Could you check a few things on this model? Use its own coordinates, in mm. A direction names the side the tool comes from. Coordinates: 2 decimals unless noted, no trailing zeros. Order: outer loops, then holes, each group sorted by start corner. A loop starts at its lowest first (then second) coordinate and runs counter-clockwise, first axis right, second up. Notation, with made-up numbers: (-24.75, 29) -> (5.25, 29) arc R18 ccw to (5.25, 46) -> close; hole circle Ø8 at (33.5, 62.5). An arc over 180 degrees is marked (long way). Use a Markdown table: item, result. Add a question column.
1) If we section it at A-A (y = -19.5): Give the number of separate pieces and of enclosed holes in the cut face, plus the area to 3 significant figures.
2) Will these pins go through, and if not, where does the flat tip stop? pin 1 Ø7.5 at (y, z) = (-16.5, 23) entering from -X; pin 2 Ø6 at (x, y) = (-173, -19.5) entering from +Z; pin 3 Ø7.5 at (y, z) = (-20, 35.5) entering from +X.
3) Thinking about a two-plate mould opening in X: for faces 4 (the cylindrical face through (-177.996, -19.312, 9.535)), 5 (the flat face through (-194, -18, 12)), 6 (the flat face through (-178.5, -20, 31)), which applies, +X half, -X half, draft (parallel to the pull), parting line (faces both ways), or undercut?
4) If I drill on L1, parallel to Y at x = -180, z = 45; L2, parallel to X at y = -24.5, z = 24; L3, parallel to Y at x = -173, z = 8, over which ranges is the centre line in solid material (lowest first)? Write a range as [from, to].
5) If we section it at C-C (x = -173): Write out the boundary of the cut face in (y, z), plus the area to 3 significant figures.
6) If we section it at D-D (z = 38): Write out the boundary of the cut face in (x, y).
7) If we section it at B-B (z = 45): Write out the boundary of the cut face in (x, y).
8) Which directions (+Z, -Z, +X, -X, +Y, -Y) give clear straight access to the entire face, cutting with the end or side of a thin tool? Please do faces 1 (the cylindrical face through (-181.458, -19.379, 47.747)), 2 (the flat face through (-171, -17, 7)), 3 (the flat face through (-187.5, -20, 35)).
```python
from build123d import *

# Parameters (mm, degrees)
SKETCH_1_W                   = 15
SKETCH_1_H                   = 15
EXTRUDE_1_DEPTH              = 50
SKETCH_2_W                   = 3
SKETCH_2_H                   = 15
CUT_EXTRUDE_1_DEPTH          = 30
SKETCH_3_W                   = 10
SKETCH_3_H                   = 15
EXTRUDE_2_DEPTH              = 12
HOLE_WIZARD_M5_2_D           = 5.3
HOLE_WIZARD_M5_2_CBORE_D     = 10
HOLE_WIZARD_M5_2_CBORE_DEPTH = 5
CUT_EXTRUDE_2_REACH          = 64.081
SKETCH_8_R                   = 2.75
M5X0_8_1_D                   = 4.2


with BuildPart() as part:
    # 草图1 → 凸台-拉伸1 (new body)
    with BuildSketch(Plane.XY):
        with Locations((-186, -19.5)):
            Rectangle(SKETCH_1_W, SKETCH_1_H)
    extrude(amount=EXTRUDE_1_DEPTH)

    # 草图2 → 切除-拉伸1 (cut)
    with BuildSketch(Plane.XY.offset(50)):
        with Locations((-186, -19.5)):
            Rectangle(SKETCH_2_W, SKETCH_2_H)
    extrude(amount=-CUT_EXTRUDE_1_DEPTH, mode=Mode.SUBTRACT)

    # 草图3 → 凸台-拉伸2 (add)
    with BuildSketch(Plane(origin=(0, 0, 0), x_dir=(-1, 0, 0), z_dir=(0, 0, -1))):
        with Locations((173.5, -19.5)):
            Rectangle(SKETCH_3_W, SKETCH_3_H)
        with Locations((198.5, -19.5)):
            Rectangle(SKETCH_3_W, SKETCH_3_H)
    extrude(amount=-EXTRUDE_2_DEPTH)

    # M5 凹头盖螺钉的柱形沉头孔2 (through all)
    with Locations(Plane.XY.offset(12)):
        with Locations((-199, -19.5), (-173, -19.5)):
            CounterBoreHole(HOLE_WIZARD_M5_2_D / 2, HOLE_WIZARD_M5_2_CBORE_D / 2, HOLE_WIZARD_M5_2_CBORE_DEPTH)

    # 草图8 → 切除-拉伸2 (cut, up to next)
    with BuildSketch(Plane(origin=(-178.5, 0, 0), x_dir=(0, 0, -1), z_dir=(1, 0, 0)), mode=Mode.PRIVATE) as cut_extrude_2_sk1:
        with Locations((-45, -19.5)):
            Circle(SKETCH_8_R)
    cut_extrude_2_tool1 = extrude(cut_extrude_2_sk1.sketch, amount=-CUT_EXTRUDE_2_REACH, mode=Mode.PRIVATE) & part.part
    add(cut_extrude_2_tool1.solids().sort_by_distance((-178.5, -19.5, 45))[0], mode=Mode.SUBTRACT)

    # M5x0.8 螺纹孔1 (through all)
    with Locations(Plane(origin=(-187.5, 0, 0), x_dir=(0, 0, -1), z_dir=(1, 0, 0))):
        with Locations((-45, -19.5)):
            Hole(M5X0_8_1_D / 2)


solid = part.part
```
Answer sheet:
| question | item | result |
|---|---|---|
| 1 | separate pieces | 5 |
| 1 | enclosed holes | 0 |
| 1 | area | 673 mm2 |
| 2 | pin 1 | x = -193.5 |
| 2 | pin 2 | z = 7 |
| 2 | pin 3 | x = -178.5 |
| 3 | face 4 | undercut |
| 3 | face 5 | draft |
| 3 | face 6 | +X half |
| 4 | L1 | [-27, -22.25], [-16.75, -12] |
| 4 | L2 | [-193.5, -187.5], [-184.5, -178.5] |
| 4 | L3 | [-27, -24.5], [-14.5, -12] |
| 5 | outline | (-27, 0) -> (-22.15, 0) -> (-22.15, 7) -> (-24.5, 7) -> (-24.5, 12) -> (-27, 12) -> close; (-16.85, 0) -> (-12, 0) -> (-12, 12) -> (-14.5, 12) -> (-14.5, 7) -> (-16.85, 7) -> close |
| 5 | area | 92.9 mm2 |
| 6 | outline | (-193.5, -27) -> (-187.5, -27) -> (-187.5, -12) -> (-193.5, -12) -> close; (-184.5, -27) -> (-178.5, -27) -> (-178.5, -12) -> (-184.5, -12) -> close |
| 7 | outline | (-193.5, -27) -> (-187.5, -27) -> (-187.5, -21.6) -> (-193.5, -21.6) -> close; (-193.5, -17.4) -> (-187.5, -17.4) -> (-187.5, -12) -> (-193.5, -12) -> close; (-184.5, -27) -> (-178.5, -27) -> (-178.5, -22.25) -> (-184.5, -22.25) -> close; (-184.5, -16.75) -> (-178.5, -16.75) -> (-178.5, -12) -> (-184.5, -12) -> close |
| 8 | face 1 | +X |
| 8 | face 2 | +Z |
| 8 | face 3 | +Z, +Y, -Y |
